CAD build for the part. Positions are in the model's coordinates, mm. A direction names the side the tool comes from. Coordinates: 2 decimals unless noted, no trailing zeros. Write each loop counter-clockwise with the first axis right and the second up, starting at its lowest first coordinate (ties: lowest second). Pieces come first, ordered by that corner, then holes.
```python
from build123d import *

# Parameters (mm, degrees)
BOSS_EXTRUDE3_DEPTH     = 20
BOSS_EXTRUDE5_DEPTH     = 1
SKETCH18_W              = 6.8
SKETCH18_H              = 5
CUT_EXTRUDE3_DEPTH      = 3
SKETCH25_R              = 8.5
BOSS_EXTRUDE6_DEPTH     = 2.5
SKETCH26_R              = 9.5
BOSS_EXTRUDE7_DEPTH     = 1
BOSS_EXTRUDE11_DEPTH    = 4
CUT_EXTRUDE7_DEPTH      = 4
SKETCH35_R              = 3.5
BOSS_EXTRUDE12_DEPTH    = 2
SKETCH36_R              = 0.8
CUT_EXTRUDE8_DEPTH      = 10.5
CUT_EXTRUDE8_DEPTH_BACK = 10.5
CUT_EXTRUDE9_DEPTH      = 6.5
CUT_EXTRUDE10_DEPTH     = 5
CUT_EXTRUDE11_DEPTH     = 19


with BuildPart() as part:
    # Sketch5 → Boss-Extrude3 (new body)
    with BuildSketch(Plane(origin=(0, 0, 0), x_dir=(1, 0, 0), z_dir=(0, 1, 0))):
        with BuildLine():
            Line((-3.983111349, -7), (3.983111349, -7))
            ThreePointArc((3.983111349, -7), (8, 0), (3.983111349, 7))
            Line((3.983111349, 7), (-3.983111349, 7))
            ThreePointArc((-3.983111349, 7), (-8, 0), (-3.983111349, -7))
        make_face()
        with BuildLine():
            Line((-3.4, -5), (3.4, -5))
            ThreePointArc((3.4, -5), (6, 0), (3.4, 5))
            Line((3.4, 5), (-3.4, 5))
            ThreePointArc((-3.4, 5), (-6, 0), (-3.4, -5))
        make_face(mode=Mode.SUBTRACT)
    extrude(amount=BOSS_EXTRUDE3_DEPTH)

    # Sketch7 → Boss-Extrude5 (add)
    with BuildSketch(Plane(origin=(0, 0, 0), x_dir=(1, 0, 0), z_dir=(0, 1, 0))):
        with BuildLine():
            Line((3.983111349, 7), (-3.983111349, 7))
            ThreePointArc((-3.983111349, 7), (-8, 0), (-3.983111349, -7))
            Line((-3.983111349, -7), (3.983111349, -7))
            ThreePointArc((3.983111349, -7), (8, 0), (3.983111349, 7))
        make_face()
    extrude(amount=BOSS_EXTRUDE5_DEPTH)

    # Sketch18 → Cut-Extrude3 (cut, through all)
    with BuildSketch(Plane.XY.offset(-5)):
        with Locations((0, 3.5)):
            Rectangle(SKETCH18_W, SKETCH18_H)
    extrude(amount=-CUT_EXTRUDE3_DEPTH, mode=Mode.SUBTRACT)

    # Sketch25 → Boss-Extrude6 (add, symmetric)
    with BuildSketch(Plane(origin=(0, 10, 0), x_dir=(1, 0, 0), z_dir=(0, 1, 0))):
        Circle(SKETCH25_R)
        with BuildLine():
            Line((3.983111349, 7), (-3.983111349, 7))
            ThreePointArc((-3.983111349, 7), (-8, 0), (-3.983111349, -7))
            Line((-3.983111349, -7), (3.983111349, -7))
            ThreePointArc((3.983111349, -7), (8, 0), (3.983111349, 7))
        make_face(mode=Mode.SUBTRACT)
    extrude(amount=BOSS_EXTRUDE6_DEPTH, both=True)

    # Sketch26 → Boss-Extrude7 (add)
    with BuildSketch(Plane(origin=(0, 12.5, 0), x_dir=(1, 0, 0), z_dir=(0, 1, 0))):
        Circle(SKETCH26_R)
        with BuildLine():
            Line((3.983111349, 7), (-3.983111349, 7))
            ThreePointArc((-3.983111349, 7), (-8, 0), (-3.983111349, -7))
            Line((-3.983111349, -7), (3.983111349, -7))
            ThreePointArc((3.983111349, -7), (8, 0), (3.983111349, 7))
        make_face(mode=Mode.SUBTRACT)
    extrude(amount=BOSS_EXTRUDE7_DEPTH)

    # Sketch32 → Boss-Extrude11 (add)
    with BuildSketch(Plane.XZ):
        with BuildLine():
            Line((-1.732050808, 1), (1.732050808, 1))
            ThreePointArc((1.732050808, 1), (0, -2), (-1.732050808, 1))
        make_face()
    extrude(amount=BOSS_EXTRUDE11_DEPTH)

    # Sketch34 → Cut-Extrude7 (cut)
    with BuildSketch(Plane.XZ.offset(4)):
        with BuildLine():
            Line((-1.118033989, 1), (1.118033989, 1))
            ThreePointArc((1.118033989, 1), (0, -1.5), (-1.118033989, 1))
        make_face()
    extrude(amount=-CUT_EXTRUDE7_DEPTH, mode=Mode.SUBTRACT)

    # Sketch35 → Boss-Extrude12 (add)
    with BuildSketch(Plane.XZ):
        Circle(SKETCH35_R)
        with BuildLine():
            Line((-1.118033989, 1), (1.118033989, 1))
            ThreePointArc((1.118033989, 1), (0, -1.5), (-1.118033989, 1))
        make_face(mode=Mode.SUBTRACT)
    extrude(amount=BOSS_EXTRUDE12_DEPTH)

    # Sketch36 → Cut-Extrude8 (cut, two sides)
    with BuildSketch(Plane(origin=(0, 0, 0), x_dir=(0, 0, -1), z_dir=(1, 0, 0))) as cut_extrude8_sk:
        with Locations((0, 17.5)):
            Circle(SKETCH36_R)
    extrude(amount=CUT_EXTRUDE8_DEPTH, mode=Mode.SUBTRACT)
    extrude(cut_extrude8_sk.sketch, amount=-CUT_EXTRUDE8_DEPTH_BACK, mode=Mode.SUBTRACT)

    # Sketch37 → Cut-Extrude9 (cut)
    with BuildSketch(Plane(origin=(0, 20, 0), x_dir=(1, 0, 0), z_dir=(0, 1, 0))):
        with BuildLine():
            Line((7.75, -1.997835367), (7.75, 1.997835367))
            ThreePointArc((7.75, 1.997835367), (8, 0), (7.75, -1.997835367))
        make_face()
        with BuildLine():
            Line((-7.75, -1.997835367), (-7.75, 1.997835367))
            ThreePointArc((-7.75, 1.997835367), (-8, 0), (-7.75, -1.997835367))
        make_face()
    extrude(amount=-CUT_EXTRUDE9_DEPTH, mode=Mode.SUBTRACT)

    # Sketch38 → Cut-Extrude10 (cut, through all)
    with BuildSketch(Plane.XZ):
        with BuildLine():
            Line((1.161895004, 1.1), (-1.161895004, 1.1))
            ThreePointArc((-1.161895004, 1.1), (0, -1.6), (1.161895004, 1.1))
        make_face()
    extrude(amount=CUT_EXTRUDE10_DEPTH, mode=Mode.SUBTRACT)

    # Sketch39 → Cut-Extrude11 (cut)
    with BuildSketch(Plane(origin=(0, 20, 0), x_dir=(1, 0, 0), z_dir=(0, 1, 0))):
        with BuildLine():
            Line((3.478078388, 5.25), (-3.478078388, 5.25))
            ThreePointArc((-3.478078388, 5.25), (-6.25, 0), (-3.478078388, -5.25))
            Line((-3.478078388, -5.25), (3.478078388, -5.25))
            ThreePointArc((3.478078388, -5.25), (6.25, 0), (3.478078388, 5.25))
        make_face()
        with BuildLine():
            Line((-3.4, 5), (3.4, 5))
            ThreePointArc((3.4, 5), (6, 0), (3.4, -5))
            Line((3.4, -5), (-3.4, -5))
            ThreePointArc((-3.4, -5), (-6, 0), (-3.4, 5))
        make_face(mode=Mode.SUBTRACT)
    extrude(amount=-CUT_EXTRUDE11_DEPTH, mode=Mode.SUBTRACT)


solid = part.part
```
Item 1: Saw through at A-A, the plane y = 17.5. Write the cut outline in (x, z).
Item 2: Flat gauge pins, fed straight in: pin 1 Ø5 at (x, y) = (-2, 5.5) entering from +Z; pin 2 Ø1 at (x, y) = (0.5, -1) entering from -Z; pin 3 Ø5 at (x, z) = (0, 0) entering from -Y; pin 4 Ø4 at (x, y) = (5.5, -0.5) entering from +Z. Where does each tip first touch, or does it go through?
Item 3: Which spindle directions (+Z, -Z, +X, -X, +Y, -Y) get a long thin tool onto all of the face, cutting with end or side? Do faces 1 (the cylindrical face through (6.342, 16.704, 4.913)), 2 (the cylindrical face through (-0.05, -1.97, -1.6)), 3 (the flat face through (0, 17, -7)), 4 (the flat face through (0, 4, 7)). Say none if no direction does.
Item 4: Wall check: line 1 along Z through (x, y) = (-1.5, 15); line 2 along Z through (x, y) = (0, -0.9); line 3 along Y through (x, z) = (3, 3.5). Give the ranges that are in metal, low to high.
Item 5: Two-plate mould, pull along X, no slides. Class faces 5 (the flat face through (7.75, 16, 0)), 6 (the flat face through (0, 1, -1)), 7 (the cylindrical face through (4.57, 10.035, -7.167)): +X half, -X half, draft (parallel to the pull), parting line (faces both ways), or undercut.
Item 6: Saw through at C-C, the plane y = 1.75. Write the cut outline in (x, z), and give its area (3 significant figures).
Item 7: Saw through at D-D, the plane z = 0. State how many separate pieces and enclosed holes the cut face has, and give its area (4 significant figures).
Working result:
1. outline: (-7.75, -2) arc R8.11 ccw to (-3.98, -7) - (3.98, -7) arc R8.11 ccw to (7.75, -2) - (7.75, -0.8) - (6.2, -0.8) arc R6.36 cw to (3.48, -5.25) - (-3.48, -5.25) arc R6.36 cw to (-6.2, -0.8) - (-7.75, -0.8) - close; (-7.75, 0.8) - (-6.2, 0.8) arc R6.36 cw to (-3.48, 5.25) - (3.48, 5.25) arc R6.36 cw to (6.2, 0.8) - (7.75, 0.8) - (7.75, 2) arc R8.11 ccw to (3.98, 7) - (-3.98, 7) arc R8.11 ccw to (-7.75, 2) - close
2. pin 1: stops at z = 8.49
2. pin 2: stops at z = -3.5
2. pin 3: stops at y = -4
2. pin 4: stops at z = 7
3. face 1: +Z, +X, +Y
3. face 2: -Y
3. face 3: -Z, +X, -X, +Y
3. face 4: +Z, +X, -X, -Y
4. line 1: z = -7 to -5.25, 5.25 to 7
4. line 2: z = -3.5 to -1.6, 1.1 to 3.5
4. line 3: y = 0 to 1
5. face 5: +X half
5. face 6: undercut
5. face 7: parting line
6. outline: (-3.98, -7) - (-3.4, -7) - (-3.4, -5.25) - (-3.48, -5.25) arc R6.36 cw to (-3.48, 5.25) - (3.48, 5.25) arc R6.36 cw to (3.48, -5.25) - (3.4, -5.25) - (3.4, -7) - (3.98, -7) arc R8.11 ccw to (3.98, 7) - (-3.98, 7) arc R8.11 ccw to start
6. area: 65.4 mm2
7. separate pieces: 3
7. enclosed holes: 0
7. area: 91.65 mm2
